from build123d import *

# Parameters (mm, degrees)
BOSS_EXTRUDE1_DEPTH      = 2
BOSS_EXTRUDE1_DEPTH_BACK = 2
SKETCH1_R                = 3
BOSS_EXTRUDE2_DEPTH      = 8
BOSS_EXTRUDE2_DEPTH_BACK = 8
SKETCH2_W                = 16
SKETCH2_H                = 4


with BuildPart() as part:
    # Sketch1 → Boss-Extrude1 (new, two sides: drawn at the far end of the back side and taken through both)
    with BuildSketch(Plane.XY.offset(-BOSS_EXTRUDE1_DEPTH_BACK)):
        with BuildLine():
            Line((-8, 0), (-8, -12))
            Line((-8, -12), (8, -12))
            Line((8, -12), (8, 0))
            ThreePointArc((8, 0), (0, 8), (-8, 0))
        make_face()
        Circle(SKETCH1_R, mode=Mode.SUBTRACT)
    extrude(amount=BOSS_EXTRUDE1_DEPTH + BOSS_EXTRUDE1_DEPTH_BACK)

    # Sketch2 → Boss-Extrude2 (add, two sides: drawn at the far end of the back side and taken through both)
    with BuildSketch(Plane.XY.offset(-BOSS_EXTRUDE2_DEPTH_BACK)):
        with Locations((0, -10)):
            Rectangle(SKETCH2_W, SKETCH2_H)
    extrude(amount=BOSS_EXTRUDE2_DEPTH + BOSS_EXTRUDE2_DEPTH_BACK)


solid = part.part
Build history of the part. All positions in model axes, mm. A direction names the side the tool comes from. Coordinates: 2 decimals unless noted, no trailing zeros. Order: outer loops, then holes, each group sorted by start corner. A loop starts at its lowest first (then second) coordinate and runs counter-clockwise, first axis right, second up. Notation, with made-up numbers: (-11, -9) - (37, -9) arc R23 ccw to (37, 22) - close; hole circle Ø3 at (-19, -12.75). An arc over 180 degrees is marked (long way). Write item = value, one per line. Start each with the question number.
1) Flat gauge pins, fed straight in: pin 1 Ø6.5 at (x, z) = (-0.5, -4) entering from +Y; pin 2 Ø1.8 at (x, z) = (0.5, 6) entering from +Y; pin 3 Ø6 at (x, y) = (1, 5) entering from +Z; pin 4 Ø1.5 at (x, y) = (-1, -2.5) entering from -Z. Where does each tip first touch, or does it go through?
2) Two-plate mould, pull along Y, no slides. Class faces 1 (the face through (-3, 0, 0)), 2 (the face through (-0.1, -3.4, -2)), 3 (the face through (0, -8, 5)): pulls with the +Y half, pulls with the -Y half, needs draft (parallel to the pull), parting line crosses it, or undercut.
3) Saw through at B-B on y = -1. Write the cut outline in (x, z).
4) Saw through at D-D on x = 2.5. Write the cut outline in (y, z), then the cut area to 3 significant figures.
5) Wall check: line 1 along Y through (x, z) = (0, 0.95); line 2 along Z through (x, y) = (-1.25, 6); line 3 along Y through (x, z) = (2.75, 1.5). Give the ranges that are in metal, low to high. Write a range as from..to.
6) Saw through at C-C on z = 1.5. Write the cut outline in (x, y).
7) 3-axis set-ups, long thin cutter, end or side, ignore diameter. For faces 4 (the face through (-0.1, -3.4, 2)), 5 (the face through (0, -8, -5)), 6 (the face through (8, -7, 0)): which of +Z, -Z, +X, -X, +Y, -Y reach the whole face in a straight line?
8) Saw through at A-A on x = 0. Write the cut outline in (y, z), then the cut area to 3 significant figures.
From the geometry:
q1.pin_1 = 8
q1.pin_2 = -8
q1.pin_3 = 2
q1.pin_4 = -2
q2.face_1 = undercut
q2.face_2 = needs draft
q2.face_3 = pulls with the +Y half
q3.outline = (-8, -2) - (-2.83, -2) - (-2.83, 2) - (-8, 2) - close; (2.83, -2) - (8, -2) - (8, 2) - (2.83, 2) - close
q4.outline = (-12, -8) - (-8, -8) - (-8, -2) - (-1.66, -2) - (-1.66, 2) - (-8, 2) - (-8, 8) - (-12, 8) - close; (1.66, -2) - (7.6, -2) - (7.6, 2) - (1.66, 2) - close
q4.area = 113 mm^2
q5.line_1 = -12..-3, 3..8
q5.line_2 = -2..2
q5.line_3 = -12..-1.2, 1.2..7.51
q6.outline = (-8, -12) - (8, -12) - (8, 0) arc R8 ccw to (-8, 0) - close; hole circle Ø6 at (0, 0)
q7.face_4 = +Z, +X, -X, +Y
q7.face_5 = -Z, +X, -X, +Y
q7.face_6 = +Z, -Z, +X, +Y, -Y
q8.outline = (-12, -8) - (-8, -8) - (-8, -2) - (-3, -2) - (-3, 2) - (-8, 2) - (-8, 8) - (-12, 8) - close; (3, -2) - (8, -2) - (8, 2) - (3, 2) - close
q8.area = 104 mm^2
